```python
from build123d import *

# Parameters (mm, degrees)
SKETCH_1_R          = 1.6
EXTRUDE_1_DEPTH     = 2
SKETCH_2_W          = 40
SKETCH_2_H          = 2
EXTRUDE_2_DEPTH     = 39
SKETCH_3_R          = 1.5
CUT_EXTRUDE_1_DEPTH = 66.064678839


with BuildPart() as part:
    # 草图1 → 凸台-拉伸1 (new body)
    with BuildSketch(Plane(origin=(0, 0, 0), x_dir=(1, 0, 0), z_dir=(0, 1, 0))):
        with BuildLine():
            Line((-21.958197384, -2.164323425), (-21.958197384, -29.664323425))
            Line((-21.958197384, -29.664323425), (18.041802616, -29.664323425))
            Line((18.041802616, -29.664323425), (18.041802616, -2.164323425))
            ThreePointArc((18.041802616, -2.164323425), (-1.958197384, 17.835676575), (-21.958197384, -2.164323425))
        make_face()
        with Locations(Location((-9.708197384, 10.259070334, 0), (0, 0, 270))):
            Circle(SKETCH_1_R, mode=Mode.SUBTRACT)
        with Locations(Location((-17.458197384, -3.164323425, 0), (0, 0, 270))):
            Circle(SKETCH_1_R, mode=Mode.SUBTRACT)
        with Locations(Location((-9.708197384, -16.587717183, 0), (0, 0, 270))):
            Circle(SKETCH_1_R, mode=Mode.SUBTRACT)
        with Locations(Location((5.791802616, -16.587717183, 0), (0, 0, 270))):
            Circle(SKETCH_1_R, mode=Mode.SUBTRACT)
        with Locations(Location((13.541802616, -3.164323425, 0), (0, 0, 270))):
            Circle(SKETCH_1_R, mode=Mode.SUBTRACT)
        with Locations(Location((5.791802616, 10.259070334, 0), (0, 0, 270))):
            Circle(SKETCH_1_R, mode=Mode.SUBTRACT)
        with BuildLine():
            Line((4.541802616, 3.835676575), (4.541802616, -10.164323425))
            ThreePointArc((4.541802616, -10.164323425), (-1.958197384, -16.664323425), (-8.458197384, -10.164323425))
            Line((-8.458197384, -10.164323425), (-8.458197384, 3.835676575))
            ThreePointArc((-8.458197384, 3.835676575), (-1.958197384, 10.335676575), (4.541802616, 3.835676575))
        make_face(mode=Mode.SUBTRACT)
    extrude(amount=EXTRUDE_1_DEPTH)

    # 草图2 → 凸台-拉伸2 (add)
    with BuildSketch(Plane(origin=(0, 2, 0), x_dir=(1, 0, 0), z_dir=(0, 1, 0))):
        with Locations((-1.958197384, -28.664323425)):
            Rectangle(SKETCH_2_W, SKETCH_2_H)
    extrude(amount=EXTRUDE_2_DEPTH)

    # 草图3 → 切除-拉伸1 (cut, through all)
    with BuildSketch(Plane(origin=(0, 0, 27.664323425), x_dir=(-1, 0, 0), z_dir=(0, 0, -1))):
        with Locations((-13.041802616, 33)):
            Circle(SKETCH_3_R)
        with Locations((-13.041802616, 9)):
            Circle(SKETCH_3_R)
        with Locations((16.958197384, 33)):
            Circle(SKETCH_3_R)
        with Locations((16.958197384, 9)):
            Circle(SKETCH_3_R)
    extrude(amount=-CUT_EXTRUDE_1_DEPTH, mode=Mode.SUBTRACT)


solid = part.part
```
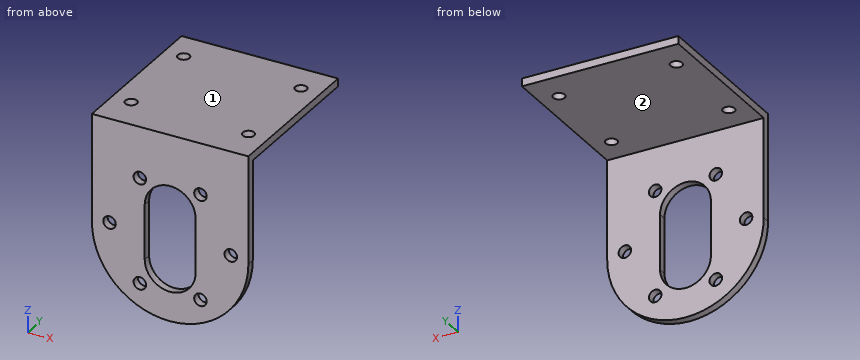
Input: part model. Units: mm. Frame: model coordinates. Face numbers are marked on the shaded views. A direction names the side the tool comes from. Round coordinates to 2 decimals unless told otherwise and drop trailing zeros. Loops run counter-clockwise (first coordinate to the right, second up) from the corner with the lowest first, then second, coordinate; pieces in that order, holes last. Notation, with made-up numbers: (-16.75, -31.5) - (31.25, -31.5) arc R13 ccw to (31.25, -24.5) - close; hole circle Ø10 at (36.25, 40.25). An arc over 180 degrees is marked (long way). One line per item, written item: value. Start each with the question number.
(1) Access query for the marked faces 1 and 2. Directions: +Z, -Z, +X, -X, +Y, -Y. A direction counts if a zero-diameter tool reaches every point of the face in a straight line with its end or side. Return the directions, or none.
(2) Section C-C, the plane x = 1.5. Return loops of the section in (y, z), plus the area to 3 significant figures.
(3) Section B-B, the plane z = 9. Return loops of the section in (x, y), plus the area to 3 significant figures.
(4) Ray query, line 1 (Y direction, x = 10.5, z = 13); line 2 (Z direction, x = -4, y = 27). Return the intervals inside material, ascending. Write a range as [from, to].
(5) Section A-A, the plane y = 33. Return loops of the section in (x, z), plus the area to 3 significant figures.
(6) Contact query for flat-ended pins moving along their axis: P1, Ø5, axis at x = -9.71, z = -10.26, coming from the +Y side; P2, Ø5, axis at x = -10.5, y = 18.5, coming from the -Z side; P3, Ø1.6, axis at y = 1.5, z = 0, coming from the -X side. Output: stop coordinate, or through.
(7) Section D-D, the plane x = -12. Return loops of the section in (y, z).
Results below:
1. face 1: +Z, +X, -X, +Y, -Y
1. face 2: -Z, +X, -X, +Y
2. outline: (0, -17.53) - (2, -17.53) - (2, -9.34) - (0, -9.34) - close; (0, 15.67) - (2, 15.67) - (2, 27.66) - (41, 27.66) - (41, 29.66) - (0, 29.66) - close
2. area: 122 mm^2
3. outline: (-21.96, 0) - (-8.46, 0) - (-8.46, 2) - (-21.96, 2) - close; (4.54, 0) - (18.04, 0) - (18.04, 2) - (4.54, 2) - close
3. area: 54.0 mm^2
4. line 1: [0, 2]
4. line 2: [27.66, 29.66]
5. outline: (-21.96, 27.66) - (-18.46, 27.66) - (-18.46, 29.66) - (-21.96, 29.66) - close; (-15.46, 27.66) - (11.54, 27.66) - (11.54, 29.66) - (-15.46, 29.66) - close; (14.54, 27.66) - (18.04, 27.66) - (18.04, 29.66) - (14.54, 29.66) - close
5. area: 68.0 mm^2
6. P1: y = 2
6. P2: z = 27.66
6. P3: x = -21.91
7. outline: (0, -15.13) - (2, -15.13) - (2, 27.66) - (41, 27.66) - (41, 29.66) - (0, 29.66) - close
